Can you work these out from the model? Positions are in its coordinate system, mm. A direction names the side the tool comes from. Round coordinates to 2 decimals unless told otherwise and drop trailing zeros. Loops run counter-clockwise (first coordinate to the right, second up) from the corner with the lowest first, then second, coordinate; pieces in that order, holes last. Notation, with made-up numbers: (-19, 24.25) -> (2, 24.25) arc R30 cw to (2, 61.25) -> close; hole circle Ø3 at (6.5, 3). An arc over 180 degrees is marked (long way). Answer as a JSON object with one key per item and string values.
Autodesk Fusion 360 part; units mm, degrees
sketch "Sketch1" plane through (0, 0, 0) normal (1, 0, 0) x (0, 0, -1)
  line L0 (0, 0) -> (40, 0)
  line L1 (40, 0) -> (40, 25)
  line L2 (40, 25) -> (0, 25)
  line L3 (0, 25) -> (0, 0)
  circle A0 centre (35, 20) radius 2
  circle A1 centre (5, 5) radius 2
  line L4 (10, 16) -> (30, 16)
  arc A2 (30, 7) -> (30, 16) centre (30, 11.5) ccw
  line L5 (30, 7) -> (10, 7)
  arc A3 (10, 16) -> (10, 7) centre (10, 11.5) ccw
  dimension "d1" = 40
  dimension "d2" = 25
  dimension "d3" = 4
  dimension "d4" = 4
  dimension "d5" = 5
  dimension "d7" = 35
  dimension "d8" = 5
  dimension "d9" = 35
  dimension "d10" = 9
  dimension "d11" = 20
  dimension "d12" = 7
  dimension "d14" = 10
extrude "Extrude1" add sketch "Sketch1" along normal blind 5
Q1. I want a section at B-B, the plane z = -17. Write out the boundary of the cut face in (x, y), then the cut area to 3 significant figures.
Determined:
{"outline": "(0, 0) -> (5, 0) -> (5, 7) -> (0, 7) -> close; (0, 16) -> (5, 16) -> (5, 25) -> (0, 25) -> close", "area": "80.0 mm²"}
Q2. On a 3-axis mill with a long thin cutter (end or side, diameter ignored), from which of +Z, -Z, +X, -X, +Y, -Y can I reach the whole of each face in a straight line? I mean faces 4 (the cylindrical face through (2.5, 11.6, -34.5)), 5 (the flat face through (2, 0, -20)). Say none if no direction works.
Determined:
{"face 4": "+X, -X", "face 5": "+Z, -Z, +X, -X, -Y"}
Q3. I want a section at C-C, the plane x = 4.2. Write out the boundary of the cut face in (y, z), then the cut area to 3 significant figures.
Determined:
{"outline": "(0, -40) -> (25, -40) -> (25, 0) -> (0, 0) -> close; hole circle Ø4 at (5, -5); hole (7, -30) arc R4.5 ccw to (16, -30) -> (16, -10) arc R4.5 ccw to (7, -10) -> close; hole circle Ø4 at (20, -35)", "area": "731 mm²"}
Q4. If I drill on L1, parallel to Y at x = 4.2, z = -29; L2, parallel to Y at x = 2.4, z = -5; L3, parallel to Z at x = 4.5, y = 21.5, over which ranges is the centre line in solid material (lowest first)? Write a range as [from, to].
Determined:
{"L1": "[0, 7], [16, 25]", "L2": "[0, 3], [7, 25]", "L3": "[-40, -36.32], [-33.68, 0]"}
Q5. We'd pull the mould along Y, two halves only. Please class faces 1 (the flat face through (2, 7, -20)), 2 (the flat face through (0, 18, -20)), 3 (the flat face through (2, 25, -20)): pulls with the +Y half, pulls with the -Y half, needs draft (parallel to the pull), parting line crosses it, or undercut.
Determined:
{"face 1": "undercut", "face 2": "needs draft", "face 3": "pulls with the +Y half"}
Q6. I want a section at A-A, the plane y = 11.5. Write out the boundary of the cut face in (x, z), then the cut area to 3 significant figures.
Determined:
{"outline": "(0, -40) -> (5, -40) -> (5, -34.5) -> (0, -34.5) -> close; (0, -5.5) -> (5, -5.5) -> (5, 0) -> (0, 0) -> close", "area": "55.0 mm²"}
